```python
from build123d import *

# Parameters (mm, degrees)
SKETCH1_R          = 26.9875
SKETCH1_R_2        = 22.225
EXTRUDE1_DEPTH     = 4.7625
SKETCH2_R          = 25.2095
SKETCH2_R_2        = 24.003
CUT_EXTRUDE1_DEPTH = 1
CUT_EXTRUDE2_START = -1
SKETCH3_R          = 25.2095
SKETCH3_R_2        = 24.003
CUT_EXTRUDE2_DEPTH = 1
CHAMFER1_SIZE      = 0.381


with BuildPart() as part:
    # Sketch1 → Extrude1 (new body)
    with BuildSketch(Plane.XY):
        with Locations(Location((-4.538848476, -45.531959332, 0), (0, 0, 180))):
            Circle(SKETCH1_R)
        with Locations(Location((-4.538848476, -45.531959332, 0), (0, 0, 180))):
            Circle(SKETCH1_R_2, mode=Mode.SUBTRACT)
    extrude(amount=EXTRUDE1_DEPTH)

    # Sketch2 → Cut-Extrude1 (cut)
    with BuildSketch(Plane.XY.offset(4.7625)):
        with Locations((-4.538848476, -45.531959332)):
            Circle(SKETCH2_R)
        with Locations((-4.538848476, -45.531959332)):
            Circle(SKETCH2_R_2, mode=Mode.SUBTRACT)
    extrude(amount=-CUT_EXTRUDE1_DEPTH, mode=Mode.SUBTRACT)

    # Sketch3 → Cut-Extrude2 (cut)
    with BuildSketch(Plane(origin=(0, 0, 0), x_dir=(-1, 0, 0), z_dir=(0, 0, -1)).offset(CUT_EXTRUDE2_START)):
        with Locations(Location((4.538848476, -45.531959332, 0), (0, 0, 180))):
            Circle(SKETCH3_R)
        with Locations(Location((4.538848476, -45.531959332, 0), (0, 0, 180))):
            Circle(SKETCH3_R_2, mode=Mode.SUBTRACT)
    extrude(amount=CUT_EXTRUDE2_DEPTH, mode=Mode.SUBTRACT)

    # Chamfer1
    chamfer1_edges = [part.edges().sort_by_distance(p)[0] for p in [
        (22.448651524, -45.531959332, 0),
        (22.448651524, -45.531959332, 4.7625),
        (17.686151524, -45.531959332, 0),
        (17.686151524, -45.531959332, 4.7625),
    ]]
    chamfer(chamfer1_edges, length=CHAMFER1_SIZE)


solid = part.part
```
Input: part model. Units: mm. Frame: model coordinates. A direction names the side the tool comes from. Round coordinates to 2 decimals unless told otherwise and drop trailing zeros.
1) Pull-direction query (X, two-part tool) for faces 1 (the cylindrical face through (1.312, -19.186, 2.353)), 2 (the cylindrical face through (-23.587, -60.137, 4.27)), 3 (the flat face through (-28.1, -35.8, 4.762)); classes: released by +X, released by -X, zero draft, split by the parting line, or undercut.
Ans:
face 1: split by the parting line
face 2: undercut
face 3: zero draft
2) Material intervals for line 1 (X direction, y = -61, z = 4.3); line 2 (Y direction, x = -5, z = 4.2); line 3 (X direction, y = -31.5, z = 0.45), sorted ascending.
Ans:
line 1: x = -26.65 to -24.45, -22.89 to -20.5, 11.42 to 13.82, 15.37 to 17.58
line 2: y = -72.52 to -70.74, -69.53 to -67.75, -23.31 to -21.53, -20.33 to -18.55
line 3: x = -27.59 to -25.48, -24.01 to -21.77, 12.7 to 14.94, 16.4 to 18.51
3) Set-up query: faces 4 (the cylindrical face through (-22.23, -61.754, 0.507)), 5 (the flat face through (-26, -37, 0)), 6 (the cylindrical face through (-7.821, -20.537, 4.27)). Return all of +Z, -Z, +X, -X, +Y, -Y with unobstructed straight access to the full face (end or side cutting, diameter ignored); none if empty.
Ans:
face 4: -Z
face 5: -Z, +X, -X, +Y, -Y
face 6: +Z
